Check sheet for the modelled part. Datum: model origin and axes. Units: mm. Give positions to 0.01 mm unless a question says otherwise; leave off trailing zeros. Order: outer loops, then holes, each group sorted by start corner. A loop starts at its lowest first (then second) coordinate and runs counter-clockwise, first axis right, second up.
Item 1: Material ranges on line 1 along X through (y, z) = (77.5, -8.45); line 2 along Y through (x, z) = (-4, -8.7); line 3 along X through (y, z) = (43, -8.15), recorded low to high.
Item 2: Sectioned sample at C-C on x = 20. Record the boundary of the cut face in (y, z), and give its area (3 significant figures).
Item 3: Release check for a two-part mould opening along X. For faces 1 (the flat face through (61.706, 29.741, -8.154)), 2 (the flat face through (-61.32, 29.41, -8.15)), 3 (the flat face through (-41.366, 25.027, -8.154)), 4 (the flat face through (41.54, 24.82, -8.15)) record: released by +X, released by -X, zero draft, split by the parting line, or undercut.
Item 4: Sectioned sample at A-A on y = 100.5. Record the boundary of the cut face in (x, z).
Item 5: Sectioned sample at B-B on z = -7.6. Record the boundary of the cut face in (x, y), and give its area (3 significant figures).
Item 6: Gauge pin test, flat ends, axial feed: P1, Ø0.5, axis at x = -69, z = -8, coming from the +Y side; P2, Ø0.5, axis at x = -17, z = -8.5, coming from the -Y side; P3, Ø0.5, axis at y = 45, z = -8.5, coming from the +X side. Record the tip position at first contact, or that the pin passes through.
from build123d import *

# Parameters (mm, degrees)
SKETCH1_W           = 134.366
SKETCH1_H           = 135.318500012
BOSS_EXTRUDE1_DEPTH = 1.5875


with BuildPart() as part:
    # Sketch1 → Boss-Extrude1 (new body)
    with BuildSketch(Plane.XY.offset(-8.9364)):
        Polygon((-62.992, 192.0875), (62.992, 192.0875), (62.992, 187.071), (70.866, 187.071), (70.866, 192.0875), (81.407, 192.0875), (81.407, 50.8), (75.438, 50.8), (75.438, 41.429545859), (47.584469242, 17.720620478), (35.318354193, 32.131), (-35.318354193, 32.131), (-47.584469242, 17.720620478), (-75.438, 41.429545859), (-75.438, 50.8), (-81.407, 50.8), (-81.407, 192.0875), (-70.866, 192.0875), (-70.866, 187.071), (-62.992, 187.071), align=None)
        with Locations((0, 115.919250006)):
            Rectangle(SKETCH1_W, SKETCH1_H, mode=Mode.SUBTRACT)
    extrude(amount=BOSS_EXTRUDE1_DEPTH)


solid = part.part
Report:
1. line 1: x = -81.41 to -67.18, 67.18 to 81.41
1. line 2: y = 32.13 to 48.26, 183.58 to 192.09
1. line 3: x = -75.44 to 75.44
2. outline: (32.13, -8.94) - (48.26, -8.94) - (48.26, -7.35) - (32.13, -7.35) - close; (183.58, -8.94) - (192.09, -8.94) - (192.09, -7.35) - (183.58, -7.35) - close
2. area: 39.1 mm2
3. face 1: released by +X
3. face 2: released by -X
3. face 3: undercut
3. face 4: undercut
4. outline: (-81.41, -8.94) - (-67.18, -8.94) - (-67.18, -7.35) - (-81.41, -7.35) - close; (67.18, -8.94) - (81.41, -8.94) - (81.41, -7.35) - (67.18, -7.35) - close
5. outline: (-81.41, 50.8) - (-75.44, 50.8) - (-75.44, 41.43) - (-47.58, 17.72) - (-35.32, 32.13) - (35.32, 32.13) - (47.58, 17.72) - (75.44, 41.43) - (75.44, 50.8) - (81.41, 50.8) - (81.41, 192.09) - (70.87, 192.09) - (70.87, 187.07) - (62.99, 187.07) - (62.99, 192.09) - (-62.99, 192.09) - (-62.99, 187.07) - (-70.87, 187.07) - (-70.87, 192.09) - (-81.41, 192.09) - close; hole (-67.18, 48.26) - (67.18, 48.26) - (67.18, 183.58) - (-67.18, 183.58) - close
5. area: 7,880 mm2
6. P1: stops at y = 187.07
6. P2: stops at y = 32.13
6. P3: stops at x = 75.44
